Source: CAD feature listing. Evaluate the final solid. Frame: model axes, mm. Give positions to 0.01 mm unless a question says otherwise; leave off trailing zeros. Loops run counter-clockwise (first coordinate to the right, second up) from the corner with the lowest first, then second, coordinate; pieces in that order, holes last. Notation, with made-up numbers: M 68,66 L 88,66 A6 cw 88,75 Z; hole C 11.5,-35 d1. An arc over 180 degrees is marked long. Write item = value, one per line.
from build123d import *

# Parameters (mm, degrees)
SKETCH1_W           = 76.2
SKETCH1_H           = 19.05
BOSS_EXTRUDE1_DEPTH = 3.175
SKETCH2_R           = 1.27
CUT_EXTRUDE1_DEPTH  = 40.400713826
FILLET1_R           = 10.16


with BuildPart() as part:
    # Sketch1 → Boss-Extrude1 (new body)
    with BuildSketch(Plane.XY):
        Rectangle(SKETCH1_W, SKETCH1_H)
    extrude(amount=BOSS_EXTRUDE1_DEPTH)

    # Sketch2 → Cut-Extrude1 (cut, through all)
    with BuildSketch(Plane.XY.offset(3.175)):
        with Locations((24.051290482, 0)):
            Circle(SKETCH2_R)
    extrude(amount=-CUT_EXTRUDE1_DEPTH, mode=Mode.SUBTRACT)

    # Fillet1
    # the kernel refuses this fillet: 10.16 mm, written as the material it takes off along each edge
    with BuildSketch(Plane(origin=(-38.1, -9.525, -25.4), x_dir=(1, 0, 0), z_dir=(0, 0, 1)), Plane(origin=(-38.1, 9.525, -25.4), x_dir=(0, -1, 0), z_dir=(0, 0, 1))) as fillet1_piece_1:
        with BuildLine():
            CenterArc((FILLET1_R, FILLET1_R), FILLET1_R, 180, 90)
            Line((0, FILLET1_R), (0, 0))
            Line((0, 0), (FILLET1_R, 0))
        make_face()
    extrude(amount=53.975, mode=Mode.SUBTRACT)
    with BuildSketch(Plane(origin=(38.1, -9.525, -25.4), x_dir=(-1, 0, 0), z_dir=(0, 0, 1)), Plane(origin=(38.1, 9.525, -25.4), x_dir=(0, -1, 0), z_dir=(0, 0, 1))) as fillet1_piece_2:
        with BuildLine():
            CenterArc((FILLET1_R, -FILLET1_R), FILLET1_R, 90, 90)
            Line((0, -FILLET1_R), (0, 0))
            Line((0, 0), (FILLET1_R, 0))
        make_face()
    extrude(amount=53.975, mode=Mode.SUBTRACT)


solid = part.part
1. Cut plane B-B, the plane y = 6.75. Return the cut outline in (x, z) (3 decimals), then the cut area to 3 significant figures.
Derived:
outline = M -34.918,0 L 34.918,0 L 34.918,3.175 L -34.918,3.175 Z
area = 222 mm²
2. Cut plane C-C, the plane y = -6.5. Return the cut outline in (x, z) (3 decimals).
Derived:
outline = M -35.173,0 L 35.173,0 L 35.173,3.175 L -35.173,3.175 Z
3. Material intervals for probe 1 along Y at (x, z) = (28.5, 2.65); probe 2 along Y at (x, z) = (23, 1) (3 decimals); probe 3 along Y at (x, z) = (25, 1.95) (3 decimals), sorted ascending. Write a range as from..to.
Derived:
probe_1 = -9.51..9.51
probe_2 = -9.525..-0.713, 0.713..9.525
probe_3 = -9.525..-0.844, 0.844..9.525
4. Pull-direction query (Y, two-part tool) for faces 1 (the cylindrical face through (22.783, 0.056, 1.61)), 2 (the cylindrical face through (34.82, -6.84, 1.57)), 3 (the cylindrical face through (-34.82, 6.84, 1.57)); classes: +Y half, -Y half, draft (parallel to the pull), parting line (faces both ways), or undercut.
Derived:
face_1 = undercut
face_2 = -Y half
face_3 = +Y half
5. First-contact query: pin 1 Ø1.5 at (y, z) = (5, 2) entering from +X; pin 2 Ø1 at (y, z) = (1, 2) entering from +X. Flat tips, straight axial feed; report the tip coordinate or a pass-through.
Derived:
pin_1 = 36.85
pin_2 = 38.04
6. Cut plane A-A, the plane z = 1.45. Return the cut outline in (x, y) (3 decimals).
Derived:
outline = M -38.08,0 A10.16 ccw -27.94,-9.525 L 27.94,-9.525 A10.16 ccw 38.08,0 A10.16 ccw 27.94,9.525 L -27.94,9.525 A10.16 ccw Z; hole C 24.051,0 d2.54
